Here's how the part is built. I have some questions about the finished solid (model axes, mm). Face numbers are marked on the shaded views. A direction names the side the tool comes from. Round coordinates to 2 decimals unless told otherwise and drop trailing zeros. Loops run counter-clockwise (first coordinate to the right, second up) from the corner with the lowest first, then second, coordinate; pieces in that order, holes last. Notation, with made-up numbers: M -19.75,7.25 L 14.25,7.25 A29 ccw 14.25,34.25 Z; hole C 56.5,43 d5. An arc over 180 degrees is marked long. Use a Markdown table: item, result.
from build123d import *

# Parameters (mm, degrees)
BOSS_EXTRUDE1_DEPTH            = 22
BOSS_EXTRUDE1_DEPTH_BACK       = 22
BOSS_EXTRUDE3_DEPTH            = 18
BOSS_EXTRUDE3_DEPTH_BACK       = 18
SKETCH5_R                      = 4
SKETCH5_R_2                    = 2.5
CUT_EXTRUDE1_DEPTH             = 43
CUT_EXTRUDE1_DEPTH_BACK        = 43
SKETCH3_R                      = 1.5
CUT_EXTRUDE3_DEPTH             = 27
CUT_EXTRUDE3_DEPTH_BACK        = 24
CUT_EXTRUDE4_REACH             = 30.697
SKETCH7_RX                     = 8
SKETCH7_RY                     = 4.8
CUT_EXTRUDE4_DIRECTION_2_REACH = 30.697


with BuildPart() as part:
    # Sketch1 → Boss-Extrude1 (new, two sides: drawn at the far end of the back side and taken through both)
    with BuildSketch(Plane(origin=(0, 0, 0), x_dir=(1, 0, 0), z_dir=(0, 1, 0)).offset(-BOSS_EXTRUDE1_DEPTH_BACK)):
        with BuildLine():
            Line((-11.950306642, 6), (-11, 0))
            Line((-11, 0), (11, 0))
            Line((11, 0), (11.950306642, 6))
            Line((11.950306642, 6), (4, 6))
            ThreePointArc((4, 6), (0, 2), (-4, 6))
            Line((-4, 6), (-11.950306642, 6))
        make_face()
        with BuildLine():
            Line((-7.641307543, 10), (-11.950306642, 6))
            Line((-11.950306642, 6), (-4, 6))
            ThreePointArc((-4, 6), (0, 10), (4, 6))
            Line((4, 6), (11.950306642, 6))
            Line((11.950306642, 6), (7.641307543, 10))
            ThreePointArc((7.641307543, 10), (4.104557854, 12.223132826), (-1.7e-08, 13))
            ThreePointArc((-1.7e-08, 13), (-4.10455787, 12.223132819), (-7.641307543, 10))
        make_face()
        with BuildLine():
            Line((-13.058997724, 13), (-11.950306642, 6))
            Line((-11.950306642, 6), (-7.641307543, 10))
            ThreePointArc((-7.641307543, 10), (-4.10455787, 12.223132819), (-1.7e-08, 13))
            Line((-1.7e-08, 13), (-2.687473981, 13))
            Line((-2.687473981, 13), (-13.058997724, 13))
        make_face()
        with BuildLine():
            Line((7.641307543, 10), (11.950306642, 6))
            Line((11.950306642, 6), (13.058997724, 13))
            Line((13.058997724, 13), (2.687473981, 13))
            Line((2.687473981, 13), (-1.7e-08, 13))
            ThreePointArc((-1.7e-08, 13), (4.104557854, 12.223132826), (7.641307543, 10))
        make_face()
    extrude(amount=BOSS_EXTRUDE1_DEPTH + BOSS_EXTRUDE1_DEPTH_BACK)

    # Sketch5 → Boss-Extrude3 (add, two sides: drawn at the far end of the back side and taken through both)
    with BuildSketch(Plane(origin=(0, 0, 0), x_dir=(1, 0, 0), z_dir=(0, 1, 0)).offset(-BOSS_EXTRUDE3_DEPTH_BACK)):
        with Locations(Location((0, 6, 0), (0, 0, 270))):
            Circle(SKETCH5_R)
        with Locations(Location((0, 6, 0), (0, 0, 270))):
            Circle(SKETCH5_R_2, mode=Mode.SUBTRACT)
    extrude(amount=BOSS_EXTRUDE3_DEPTH + BOSS_EXTRUDE3_DEPTH_BACK)

    # Sketch3 → Cut-Extrude1 (cut, two sides: drawn at the far end of the back side and taken through both)
    with BuildSketch(Plane(origin=(0, 0, 0), x_dir=(0, 0, -1), z_dir=(1, 0, 0)).offset(-CUT_EXTRUDE1_DEPTH_BACK)):
        with Locations(Location((8, 15, 0), (0, 0, 180))):
            Circle(SKETCH3_R)
        with Locations(Location((8, -15, 0), (0, 0, 180))):
            Circle(SKETCH3_R)
    extrude(amount=CUT_EXTRUDE1_DEPTH + CUT_EXTRUDE1_DEPTH_BACK, mode=Mode.SUBTRACT)

    # Sketch6 → Cut-Extrude3 (cut, two sides: drawn at the far end of the back side and taken through both)
    with BuildSketch(Plane.XY.offset(-CUT_EXTRUDE3_DEPTH_BACK)):
        with BuildLine():
            ThreePointArc((-9, -11.5), (-7.681980515, -14.681980515), (-4.5, -16))
            Line((-4.5, -16), (4.5, -16))
            ThreePointArc((4.5, -16), (7.681980515, -14.681980515), (9, -11.5))
            Line((9, -11.5), (9, 11.5))
            ThreePointArc((9, 11.5), (7.681980515, 14.681980515), (4.5, 16))
            Line((4.5, 16), (-4.5, 16))
            ThreePointArc((-4.5, 16), (-7.681980515, 14.681980515), (-9, 11.5))
            Line((-9, 11.5), (-9, -11.5))
        make_face()
    extrude(amount=CUT_EXTRUDE3_DEPTH + CUT_EXTRUDE3_DEPTH_BACK, mode=Mode.SUBTRACT)

    # Cut-Extrude4: up to this plane
    cut_extrude4_end = Plane(origin=(-10.73081084, -22, 1.699593469), z_dir=(-0.9876883405951371, 0, 0.15643446504023473))
    # Sketch7 → Cut-Extrude4 (cut, up to the surface)
    with BuildSketch(Plane(origin=(0, 0, 0), x_dir=(0, 0, -1), z_dir=(1, 0, 0)), mode=Mode.PRIVATE) as cut_extrude4_sk1:
        with Locations(Location((0, 0), (0, 0, 90))):
            Ellipse(SKETCH7_RX, SKETCH7_RY)
    cut_extrude4_tool1 = split(extrude(cut_extrude4_sk1.sketch, amount=-CUT_EXTRUDE4_REACH, mode=Mode.PRIVATE), bisect_by=cut_extrude4_end, keep=Keep.BOTH, mode=Mode.PRIVATE)
    add(cut_extrude4_tool1.solids().sort_by_distance((0, 0, 0))[0], mode=Mode.SUBTRACT)

    # Cut-Extrude4 direction 2: up to this plane
    cut_extrude4_direction_2_end = Plane(origin=(10.73081084, -22, 1.699593469), z_dir=(-0.9876883405951371, 0, -0.15643446504023442))
    # Sketch7 → Cut-Extrude4 direction 2 (cut, up to the surface)
    with BuildSketch(Plane(origin=(0, 0, 0), x_dir=(0, 0, -1), z_dir=(1, 0, 0)), mode=Mode.PRIVATE) as cut_extrude4_direction_2_sk1:
        with Locations(Location((0, 0), (0, 0, 90))):
            Ellipse(SKETCH7_RX, SKETCH7_RY)
    cut_extrude4_direction_2_tool1 = split(extrude(cut_extrude4_direction_2_sk1.sketch, amount=CUT_EXTRUDE4_DIRECTION_2_REACH, mode=Mode.PRIVATE), bisect_by=cut_extrude4_direction_2_end, keep=Keep.BOTH, mode=Mode.PRIVATE)
    add(cut_extrude4_direction_2_tool1.solids().sort_by_distance((0, 0, 0))[0], mode=Mode.SUBTRACT)


solid = part.part
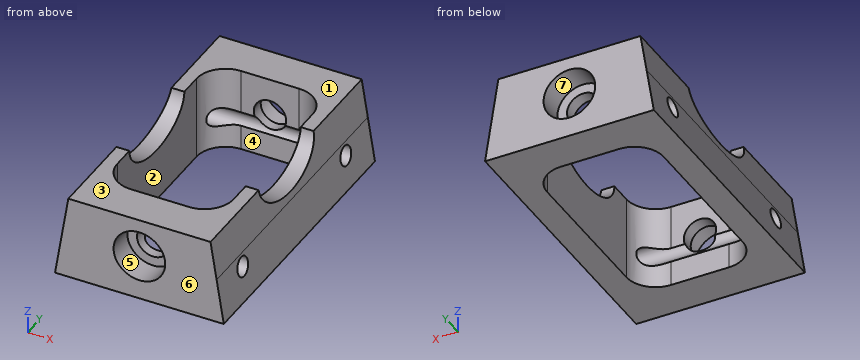
1. Imagine slicing it at A-A, the plane y = -10.5. Write out the boundary of the cut face in (x, z).
Answer sheet:
| item | result |
|---|---|
| outline | M -13.06,-13 L -9,-13 L -9,0 L -11,0 Z; M 9,-13 L 13.06,-13 L 11,0 L 9,0 Z |
2. We'd pull the mould along X, two halves only. Please class the marked faces 1 and 2: +X half, -X half, draft (parallel to the pull), parting line (faces both ways), or undercut.
Answer sheet:
| item | result |
|---|---|
| face 1 | draft |
| face 2 | undercut |
3. Imagine slicing it at D-D, the plane x = 0. Write out the boundary of the cut face in (y, z), then the cut area to 3 significant figures.
Answer sheet:
| item | result |
|---|---|
| outline | M -22,-13 L -16,-13 L -16,-9.12 A1.5 cw -16.41,-8.5 L -18,-8.5 L -18,-10 L -22,-10 Z; M -22,-2 L -18,-2 L -18,-3.5 L -16,-3.5 L -16,0 L -22,0 Z; M 16,-13 L 22,-13 L 22,-10 L 18,-10 L 18,-8.5 L 16.41,-8.5 A1.5 cw 16,-9.12 Z; M 16,-3.5 L 18,-3.5 L 18,-2 L 22,-2 L 22,0 L 16,0 Z |
| area | 71.7 mm2 |
4. For pin 1 Ø4 at (y, z) = (-4, -5.5) entering from +X; pin 2 Ø7.5 at (x, z) = (-1.5, -3.5) entering from -Y; pin 3 Ø3 at (y, z) = (-13.5, -4) entering from -X; pin 4 Ø7 at (x, z) = (0, -6) entering from -Y, each with a flat end and sliding along its axis, tell me the tip position at first contact or that it passes through.
Answer sheet:
| item | result |
|---|---|
| pin 1 | x = 12.19 |
| pin 2 | y = -22 |
| pin 3 | x = -11.87 |
| pin 4 | y = -18 |
5. Imagine slicing it at C-C, the plane x = -6.75. Write out the boundary of the cut face in (y, z).
Answer sheet:
| item | result |
|---|---|
| outline | M -22,-13 L -15.4,-13 L -15.4,-9.45 A1.5 cw -15.4,-6.55 L -15.4,0 L -22,0 Z; M 15.4,-13 L 22,-13 L 22,0 L 15.4,0 L 15.4,-6.55 A1.5 cw 15.4,-9.45 Z |
6. Imagine slicing it at B-B, the plane y = -17. Write out the boundary of the cut face in (x, z).
Answer sheet:
| item | result |
|---|---|
| outline | M -13.06,-13 L 13.06,-13 L 11,0 L -11,0 Z; hole C 0,-6 d5 |
7. Which directions (+Z, -Z, +X, -X, +Y, -Y) give clear straight access to the entire face, cutting with the end or side of a thin tool? Please do the marked faces 3, 4, 5, 6 and 7.
Answer sheet:
| item | result |
|---|---|
| face 3 | +Z, +X, -X, +Y, -Y |
| face 4 | +Z, -Z |
| face 5 | -Y |
| face 6 | +Z, -Z, +X, -X, -Y |
| face 7 | +Y |
8. I need wall thicknesses on probe 1 along Z at (x, y) = (0, -18.95); probe 2 along X at (y, z) = (19.1, -6); probe 3 along Y at (x, z) = (6, -8). Which ranges of each line are inside material? Lowest first, please. Write a range as from..to.
Answer sheet:
| item | result |
|---|---|
| probe 1 | -13..-10, -2..0 |
| probe 2 | -11.95..-4, 4..11.95 |
| probe 3 | -22..-16.5, 16.5..22 |
